from build123d import *

# Parameters (mm, degrees)
CROQUIS2_W              = 16.2
CROQUIS2_H              = 9.2
CROQUIS2_W_2            = 13.2
CROQUIS2_H_2            = 6.2
SALIENTE_EXTRUIR1_DEPTH = 6.5
CROQUIS3_W              = 16.2
CROQUIS3_H              = 12
SALIENTE_EXTRUIR2_DEPTH = 2
SALIENTE_EXTRUIR3_DEPTH = 8.1
CROQUIS5_W              = 16.2
CROQUIS5_H              = 3
SALIENTE_EXTRUIR4_DEPTH = 13
CROQUIS6_R              = 1.6
CORTAR_EXTRUIR1_DEPTH   = 3
CROQUIS7_W              = 16.2
CROQUIS7_H              = 2
SALIENTE_EXTRUIR5_DEPTH = 3
CROQUIS8_R              = 2.9
CORTAR_EXTRUIR2_DEPTH   = 0.5
REDONDEO1_R             = 1
REDONDEO2_R             = 1
REDONDEO3_R             = 2
REDONDEO4_R             = 2
REDONDEO5_R             = 3
REDONDEO6_R             = 8
CROQUIS9_W              = 13.2
CROQUIS9_H              = 6.2
SALIENTE_EXTRUIR6_DEPTH = 3.5
CROQUIS10_W             = 13.2
CROQUIS10_H             = 1.5
SALIENTE_EXTRUIR7_DEPTH = 3.5


with BuildPart() as part:
    # Croquis2 → Saliente-Extruir1 (new body)
    with BuildSketch(Plane(origin=(0, 0, 0), x_dir=(1, 0, 0), z_dir=(0, 1, 0))):
        with Locations((6.6, -3.1)):
            Rectangle(CROQUIS2_W, CROQUIS2_H)
        with Locations((6.6, -3.1)):
            Rectangle(CROQUIS2_W_2, CROQUIS2_H_2, mode=Mode.SUBTRACT)
    extrude(amount=SALIENTE_EXTRUIR1_DEPTH)

    # Croquis3 → Saliente-Extruir2 (add)
    with BuildSketch(Plane(origin=(0, 0, -1.5), x_dir=(-1, 0, 0), z_dir=(0, 0, -1))):
        with Locations((-6.6, 6)):
            Rectangle(CROQUIS3_W, CROQUIS3_H)
    extrude(amount=SALIENTE_EXTRUIR2_DEPTH)

    # Croquis4 → Saliente-Extruir3 (add)
    with BuildSketch(Plane(origin=(0, 0, -3.5), x_dir=(-1, 0, 0), z_dir=(0, 0, -1))):
        Polygon((1.5, 0), (1.5, 12), (-14.7, 12), (-14.7, 0), (-12.9, 0), (-12.9, 10), (-0.3, 10), (-0.3, 0), align=None)
    extrude(amount=SALIENTE_EXTRUIR3_DEPTH)

    # Croquis5 → Saliente-Extruir4 (add)
    with BuildSketch(Plane(origin=(0, 12, 0), x_dir=(1, 0, 0), z_dir=(0, 1, 0))):
        with Locations((6.6, 10.1)):
            Rectangle(CROQUIS5_W, CROQUIS5_H)
    extrude(amount=SALIENTE_EXTRUIR4_DEPTH)

    # Croquis6 → Cortar-Extruir1 (cut)
    with BuildSketch(Plane.XY.offset(-8.6)):
        with Locations((9.1, 20)):
            Circle(CROQUIS6_R)
    extrude(amount=-CORTAR_EXTRUIR1_DEPTH, mode=Mode.SUBTRACT)

    # Croquis7 → Saliente-Extruir5 (add)
    with BuildSketch(Plane.XY.offset(-1.5)):
        with Locations((6.6, 7.5)):
            Rectangle(CROQUIS7_W, CROQUIS7_H)
    extrude(amount=SALIENTE_EXTRUIR5_DEPTH)

    # Croquis8 → Cortar-Extruir2 (cut)
    with BuildSketch(Plane.XY.offset(-8.6)):
        with Locations((9.1, 20)):
            Circle(CROQUIS8_R)
    extrude(amount=-CORTAR_EXTRUIR2_DEPTH, mode=Mode.SUBTRACT)

    # Redondeo1
    redondeo1_edges = [part.edges().sort_by_distance(p)[0] for p in [
        (14.7, 3.25, 7.7),
        (-1.5, 3.25, 7.7),
    ]]
    fillet(redondeo1_edges, radius=REDONDEO1_R)

    # Redondeo2
    redondeo2_edges = [part.edges().sort_by_distance(p)[0] for p in [
        (6.6, 8.5, 1.5),
    ]]
    fillet(redondeo2_edges, radius=REDONDEO2_R)

    # Redondeo3
    redondeo3_edges = [part.edges().sort_by_distance(p)[0] for p in [
        (6.6, 8.5, -1.5),
    ]]
    fillet(redondeo3_edges, radius=REDONDEO3_R - 0.0001)  # a hair under: the kernel refuses the full size

    # Redondeo4
    redondeo4_edges = [part.edges().sort_by_distance(p)[0] for p in [
        (6.6, 12, -1.5),
    ]]
    fillet(redondeo4_edges, radius=REDONDEO4_R)

    # Redondeo5
    redondeo5_edges = [part.edges().sort_by_distance(p)[0] for p in [
        (6.6, 12, -8.6),
    ]]
    fillet(redondeo5_edges, radius=REDONDEO5_R)

    # Redondeo6
    redondeo6_edges = [part.edges().sort_by_distance(p)[0] for p in [
        (14.7, 25, -10.1),
        (-1.5, 25, -10.1),
    ]]
    fillet(redondeo6_edges, radius=REDONDEO6_R)

    # Croquis9 → Saliente-Extruir6 (add)
    with BuildSketch(Plane.XZ):
        with BuildLine():
            Line((13.7, 7.7), (-0.5, 7.7))
            ThreePointArc((-0.5, 7.7), (-1.207106781, 7.407106781), (-1.5, 6.7))
            Line((-1.5, 6.7), (-1.5, -11.6))
            Line((-1.5, -11.6), (0.3, -11.6))
            Line((0.3, -11.6), (0.3, -3.5))
            Line((0.3, -3.5), (12.9, -3.5))
            Line((12.9, -3.5), (12.9, -11.6))
            Line((12.9, -11.6), (14.7, -11.6))
            Line((14.7, -11.6), (14.7, 6.7))
            ThreePointArc((14.7, 6.7), (14.407106781, 7.407106781), (13.7, 7.7))
        make_face()
        with Locations((6.6, 3.1)):
            Rectangle(CROQUIS9_W, CROQUIS9_H, mode=Mode.SUBTRACT)
    extrude(amount=SALIENTE_EXTRUIR6_DEPTH)

    # Croquis10 → Saliente-Extruir7 (add)
    with BuildSketch(Plane.XZ.offset(-6.5)):
        with Locations((6.6, 0.75)):
            Rectangle(CROQUIS10_W, CROQUIS10_H)
    extrude(amount=SALIENTE_EXTRUIR7_DEPTH)


solid = part.part
The model under review builds one solid part; all positions refer to its coordinate system, in mm. A direction names the side the tool comes from. Round coordinates to 2 decimals unless told otherwise and drop trailing zeros. Write each loop counter-clockwise with the first axis right and the second up, starting at its lowest first coordinate (ties: lowest second). Pieces come first, ordered by that corner, then holes. Notation, with made-up numbers: M 0,87.5 L 53,87.5 A22 ccw 53,96.5 Z; hole C 21.5,14 d8. An arc over 180 degrees is marked long. Answer as CSV lines item,"result". Start each with the question number.
Q1. Consider section A-A, the plane z = 4.75. Give the boundary of the cut face in (x, y).
Q2. The part is to be moulded in two halves that separate along X. For faces 4 (the face through (0.781, 22.594, -10.121)), 5 (the face through (6, 5, 1.5)), 6 (the face through (6.71, 8.99, -0.81)), say which applies: +X half, -X half, draft (parallel to the pull), parting line (faces both ways), or undercut.
Q3. Wall thickness on line 1 along X through (y, z) = (9, -7.75); line 2 along Z through (x, y) = (2.5, 0.75); line 3 along X through (y, z) = (-1, 5.75): over which ranges is each line inside the solid? List them lowest first.
Q4. Consider section D-D, the plane z = -7. Give the boundary of the cut face in (x, y), then the cut area to 3 significant figures.
Q5. Clearance check with flat-ended pins moving along their axes: P1, Ø5, axis at x = 9.1, y = 20, coming from the +Z side; P2, Ø5, axis at x = 3.5, y = 18, coming from the +Z side; P3, Ø1.9, axis at x = 6, z = 5.5, coming from the +Y side; P4, Ø8, axis at x = 1.5, z = -7, coming from the -Y side. State where each tip first meets the part, or that it passes through.
Q6. Consider section B-B, the plane y = -0.5. Give the boundary of the cut face in (x, z).
Q7. Consider section C-C, the plane y = 20. Give the boundary of the cut face in (x, z).
Q8. Tool access review of faces 1 (the face through (7, 10, -7)), 2 (the face through (7, 0, 0)), 3 (the face through (6, 6.5, 7)): name each direction out of +Z, -Z, +X, -X, +Y, -Y from which nothing blocks a thin tool from reaching the whole face with its end or side.
Result set:
1,outline,"M -1.5,-3.5 L 0,-3.5 L 0,6.5 L -1.5,6.5 Z; M 13.2,-3.5 L 14.7,-3.5 L 14.7,6.5 L 13.2,6.5 Z"
2,face 4,"-X half"
2,face 5,"undercut"
2,face 6,"draft"
3,line 1,"x = -1.5 to 0.3, 12.9 to 14.7"
3,line 2,"z = -3.5 to 0, 6.2 to 7.7"
3,line 3,"x = -1.5 to 0, 13.2 to 14.7"
4,outline,"M -1.5,-3.5 L 0.3,-3.5 L 0.3,10 L 12.9,10 L 12.9,-3.5 L 14.7,-3.5 L 14.7,12.35 L -1.5,12.35 Z"
4,area,"86.6 mm²"
5,P1,"stops at z = -9.1"
5,P2,"stops at z = -8.6"
5,P3,"stops at y = 6.5"
5,P4,"stops at y = -3.5"
6,outline,"M -1.5,-11.6 L 0.3,-11.6 L 0.3,-3.5 L 12.9,-3.5 L 12.9,-11.6 L 14.7,-11.6 L 14.7,6.7 A1 ccw 13.7,7.7 L -0.5,7.7 A1 ccw -1.5,6.7 Z; hole M 0,0 L 13.2,0 L 13.2,6.2 L 0,6.2 Z"
7,outline,"M -0.92,-11.6 L 7.5,-11.6 L 7.5,-9.1 L 6.2,-9.1 L 6.2,-8.6 L -0.92,-8.6 Z; M 10.7,-11.6 L 14.12,-11.6 L 14.12,-8.6 L 12,-8.6 L 12,-9.1 L 10.7,-9.1 Z"
8,face 1,"-Z, -Y"
8,face 2,"-Y"
8,face 3,"+Z, +X, -X, +Y"
